```python
from build123d import *
from build123d.topology import SkipClean

# Parameters (mm, degrees)
SKETCH3_R           = 14
SKETCH3_R_2         = 11
SKETCH5_R           = 14
SKETCH5_R_2         = 11
BOSS_EXTRUDE1_DEPTH = 42
CUT_EXTRUDE1_START  = -95
SKETCH6_R           = 11
CUT_EXTRUDE1_DEPTH  = 95
CUT_EXTRUDE2_START  = -33
SKETCH7_R           = 11
CUT_EXTRUDE2_DEPTH  = 33


with BuildPart() as part:
    # Sweep1: sweep along a path in Sketch1
    with BuildLine(Plane.XY) as sweep1_path:
        Line((42, 0), (0, 0))
        Line((0, 0), (-42, 0))
    # Sketch3 → Sweep1 (sweep)
    with BuildSketch(Plane(origin=(32, 0, 0), x_dir=(0, 0, -1), z_dir=(1, 0, 0))):
        Circle(SKETCH3_R)
        Circle(SKETCH3_R_2, mode=Mode.SUBTRACT)
    sweep(path=sweep1_path.line)

    # Sketch5 → Boss-Extrude1 (add)
    with BuildSketch(Plane(origin=(0, 0, 0), x_dir=(1, 0, 0), z_dir=(0, 1, 0))):
        with Locations(Location((0, 0, 0), (0, 0, 270))):
            Circle(SKETCH5_R)
        with Locations(Location((0, 0, 0), (0, 0, 270))):
            Circle(SKETCH5_R_2, mode=Mode.SUBTRACT)
    extrude(amount=BOSS_EXTRUDE1_DEPTH)

    # Sketch6 → Cut-Extrude1 (cut)
    with SkipClean():  # the faces are left unmerged after this step: merging them gives an invalid solid
        with BuildSketch(Plane(origin=(42, 0, 0), x_dir=(0, 0, -1), z_dir=(1, 0, 0)).offset(CUT_EXTRUDE1_START)):
            Circle(SKETCH6_R)
        extrude(amount=CUT_EXTRUDE1_DEPTH, mode=Mode.SUBTRACT)

    # Sketch7 → Cut-Extrude2 (cut)
    with SkipClean():  # the faces are left unmerged after this step: merging them gives an invalid solid
        with BuildSketch(Plane(origin=(0, 42, 0), x_dir=(1, 0, 0), z_dir=(0, 1, 0)).offset(CUT_EXTRUDE2_START)):
            with Locations(Location((0, 0, 0), (0, 0, 270))):
                Circle(SKETCH7_R)
        extrude(amount=CUT_EXTRUDE2_DEPTH, mode=Mode.SUBTRACT)


solid = part.part
```
The listing builds one solid part. Answer for the finished solid, in the listing's coordinates (mm). A direction names the side the tool comes from. Round coordinates to 2 decimals unless told otherwise and drop trailing zeros. Order: outer loops, then holes, each group sorted by start corner. A loop starts at its lowest first (then second) coordinate and runs counter-clockwise, first axis right, second up. Notation, with made-up numbers: (-8, -7.75) -> (30, -7.75) arc R22 cw to (30, 29.25) -> close; hole circle Ø7 at (40.5, -32). An arc over 180 degrees is marked (long way). Answer as CSV lines item,"result". Start each with the question number.
(1) The part is cut by section B-B (x = 0). Determine the outline of the cut face in (y, z), then the cut area to 3 significant figures.
(2) For a pull along Y with two mould halves and no side action, classify faces 1 (the face through (-0.588, -10.906, 1.432)), 2 (the face through (-0.59, -13.88, 1.82)), 3 (the face through (-42, 9.3, 6.2)) as +Y half, -Y half, draft (parallel to the pull), parting line (faces both ways), or undercut.
(3) The part is cut by section D-D (y = 34). Determine the outline of the cut face in (x, z), then the cut area to 3 significant figures.
(4) Find the intervals of material crossed by probe 1 along X at (y, z) = (24, 0), in increasing order. Write a range as from..to.
(5) The part is cut by section A-A (z = 0). Determine the outline of the cut face in (x, y).
(6) A tool of negligible diameter and unlimited length cuts with its end or side. For faces 4 (the face through (-9.3, 42, 6.2)), 5 (the face through (0.616, 25.373, -13.986)), from which of +Z, -Z, +X, -X, +Y, -Y can it reach the whole face along a straight path? Write none if from no direction.
(7) Flat-ended cylindrical pins translate along their axes: pin 1 Ø2 at (x, z) = (1, 9) entering from +Y; pin 2 Ø4 at (x, y) = (-24, 10) entering from -Z; pin 3 Ø1.5 at (x, y) = (17, 2) entering from -Z. Find the tip coordinate at first contact, or state that the pin passes through.
(8) The part is cut by section C-C (y = -7). Determine the outline of the cut face in (x, z).
Evaluation:
1,outline,"(0, -14) -> (42, -14) -> (42, -11) -> (8.66, -11) arc R14 ccw to (9, -10.72) -> (9, -6.32) arc R11 cw (long way) to (9, 6.32) -> (9, 10.72) arc R14 ccw to (8.66, 11) -> (42, 11) -> (42, 14) -> (0, 14) arc R14 ccw to start"
1,area,"395 mm²"
2,face 1,"undercut"
2,face 2,"parting line"
2,face 3,"draft"
3,outline,"circle Ø28 at (0, 0); hole circle Ø22 at (0, 0)"
3,area,"236 mm²"
4,probe 1,"-14..-11, 11..14"
5,outline,"(-42, -14) -> (42, -14) -> (42, -11) -> (-42, -11) -> close; (-42, 11) -> (-11, 11) -> (-11, 42) -> (-14, 42) -> (-14, 14) -> (-42, 14) -> close; (11, 11) -> (42, 11) -> (42, 14) -> (14, 14) -> (14, 42) -> (11, 42) -> close"
6,face 4,"+Z, -Z, +X, -X, +Y"
6,face 5,"+Y"
7,pin 1,"y = 9"
7,pin 2,"z = -11.49"
7,pin 3,"z = -13.94"
8,outline,"(-42, -12.12) -> (42, -12.12) -> (42, -8.49) -> (-42, -8.49) -> close; (-42, 8.49) -> (42, 8.49) -> (42, 12.12) -> (-42, 12.12) -> close"
